Source: CAD feature listing. Evaluate the final solid. Frame: model axes, mm. A direction names the side the tool comes from. Round coordinates to 2 decimals unless told otherwise and drop trailing zeros. Order: outer loops, then holes, each group sorted by start corner. A loop starts at its lowest first (then second) coordinate and runs counter-clockwise, first axis right, second up. Notation, with made-up numbers: (34.5, -4) - (43.5, -4) arc R28 ccw to (43.5, 16) - close; hole circle Ø7 at (69, 59.5). An arc over 180 degrees is marked (long way). Use one line per item in the form item = value. Start each with the question number.
Q1. Cut plane C-C, the plane y = -1.25. Give the number of separate pieces and of enclosed holes in the cut face, and give its area (3 significant figures).
Q2. Cut plane A-A, the plane z = 3.5. Return the cut outline in (x, y), and give its area (3 significant figures).
Q3. Cut plane B-B, the plane x = -13. Return the cut outline in (y, z), and give its area (3 significant figures).
Q4. Ray query, line 1 (X direction, y = -2, z = 3); line 2 (Z direction, x = -2.5, y = -6.75); line 3 (X direction, y = -5.25, z = 1). Return the intervals inside material, ascending. Write a range as [from, to].
Q5. Set-up query: faces 1 (the cylindrical face through (11.616, -1.252, 3.556)), 2 (the cylindrical face through (0.18, -8.38, 4.16)), 3 (the cylindrical face through (-10.57, -5.47, 6.05)), 4 (the cylindrical face through (10.58, -5.47, 0.32)). Return all of +Z, -Z, +X, -X, +Y, -Y with unobstructed straight access to the full face (end or side cutting, diameter ignored); none if empty.
Q6. Cut plane D-D, the plane x = -7. Return the cut outline in (y, z).
Q7. Draft query along X for faces 5 (the cylindrical face through (-9.525, -5.67, 3.211)), 6 (the flat face through (-14.2, -2.54, 2.5)), 7 (the cylindrical face through (0.131, -5.968, 1.002)). Return one class per face: released by +X, released by -X, zero draft, split by the parting line, or undercut.
Q8. Pin query (flat end, axial travel): pin 1 Ø1.5 at (y, z) = (-3.5, 4.5) entering from -X; pin 2 Ø2 at (x, z) = (-12.827, 3.175) entering from -Y; pin 3 Ø3 at (y, z) = (-8.5, 3.5) entering from -X; pin 4 Ø4 at (x, y) = (2, -5.5) entering from +Z. Return the tip coordinate at first contact, or that it passes through.
from build123d import *

# Parameters (mm, degrees)
F1_DEPTH = 6.35
F2_DEPTH = 2.54
F3_R     = 1.27
F4_DEPTH = 25.4
F7_DEPTH = 10.16
F8_R     = 0.508
F9_SIZE  = 0.508


with BuildPart() as f1:
    # F0 (on Top) → F1 (new body)
    with BuildSketch(Plane.XY):
        with BuildLine():
            ThreePointArc((8.382, 0), (0, -8.382), (-8.382, 0))
            Line((-8.382, 0), (-17.272, 0))
            Line((-17.272, 0), (-17.272, -2.54))
            Line((-17.272, -2.54), (-15.24, -2.54))
            ThreePointArc((-15.24, -2.54), (-8.8418597658, -9.1442704985), (0, -11.6689691252))
            ThreePointArc((0, -11.6689691252), (8.8418597658, -9.1442704985), (15.24, -2.54))
            Line((15.24, -2.54), (17.272, -2.54))
            Line((17.272, -2.54), (17.272, 0))
            Line((17.272, 0), (8.382, 0))
        make_face()
    extrude(amount=F1_DEPTH)

    # F0 (on Top) → F2 (join)
    with BuildSketch(Plane.XY):
        with BuildLine():
            ThreePointArc((5.969, 0), (0, -5.969), (-5.969, 0))
            Line((-5.969, 0), (-8.382, 0))
            ThreePointArc((-8.382, 0), (0, -8.382), (8.382, 0))
            Line((8.382, 0), (5.969, 0))
        make_face()
    extrude(amount=F2_DEPTH)

    # F3 (on face) → F4 (cut)
    with BuildSketch(Plane(origin=(0, 0, 0), x_dir=(-1, 0, 0), z_dir=(0, 1, 0))):
        with Locations((-12.827, 3.175)):
            Circle(F3_R)
        with Locations((12.827, 3.175)):
            Circle(F3_R)
    extrude(amount=-F4_DEPTH, mode=Mode.SUBTRACT)

    # F6 (on offset) → F7 (cut)
    with BuildSketch(Plane(origin=(0, -12.7, 0), x_dir=(-1, 0, 0), z_dir=(0, 1, 0))):
        with BuildLine():
            ThreePointArc((12.7267177602, -0.1254768553), (15.1261381042, 0.8049434652), (16.129, 3.175))
            ThreePointArc((16.129, 3.175), (15.1883800681, 5.483048564), (12.9024172176, 6.4761386283))
            ThreePointArc((12.9024172176, 6.4761386283), (9.5261688447, 3.2628503518), (12.7267177602, -0.1254768553))
        make_face()
        with BuildLine():
            ThreePointArc((-12.7793536698, -0.1266562249), (-10.4753482207, 0.8570401408), (-9.525, 3.175))
            ThreePointArc((-9.525, 3.175), (-10.4531379965, 5.4702087461), (-12.7157832758, 6.4751264885))
            ThreePointArc((-12.7157832758, 6.4751264885), (-16.128846925, 3.2067943984), (-12.7793536698, -0.1266562249))
        make_face()
        with BuildLine():
            ThreePointArc((-12.7793536698, -0.1266562249), (-16.128846925, 3.2067943984), (-12.7157832758, 6.4751264885))
            Line((-12.7157832758, 6.4751264885), (-20.0003515929, 7.2803031653))
            Line((-20.0003515929, 7.2803031653), (-20.0003515929, -2.0043456461))
            Line((-20.0003515929, -2.0043456461), (-12.7793536698, -0.1266562249))
        make_face()
        with BuildLine():
            ThreePointArc((12.9024172176, 6.4761386283), (15.1883800681, 5.483048564), (16.129, 3.175))
            ThreePointArc((16.129, 3.175), (15.1261381042, 0.8049434652), (12.7267177602, -0.1254768553))
            Line((12.7267177602, -0.1254768553), (20.6403024495, -1.1550099589))
            Line((20.6403024495, -1.1550099589), (20.6403024495, 7.2800177149))
            Line((20.6403024495, 7.2800177149), (12.9024172176, 6.4761386283))
        make_face()
    extrude(amount=F7_DEPTH, mode=Mode.SUBTRACT)

    # F8
    f8_edges = [f1.edges().sort_by_distance(p)[0] for p in [
        (-11.920039, -4.675696, 6.35),
        (-11.920039, -4.675696, 0),
        (11.920039, -4.675696, 6.35),
        (11.920039, -4.675696, 0),
    ]]
    fillet(f8_edges, radius=F8_R)

    # F9
    f9_edges = [f1.edges().sort_by_distance(p)[0] for p in [
        (0, -5.969, 2.54),
        (7.1755, 0, 2.54),
        (-7.1755, 0, 2.54),
    ]]
    chamfer(f9_edges, length=F9_SIZE)


solid = f1.part
Completed:
q1.separate_pieces = 2
q1.enclosed_holes = 2
q1.area = 116 mm2
q2.outline = (-17.27, -2.54) - (-14.05, -2.54) - (-14.05, 0) - (-17.27, 0) - close; (-11.6, -2.54) - (-9.54, -2.54) - (-9.54, -8.7) arc R17.78 ccw to (0, -11.67) arc R17.78 ccw to (9.54, -8.7) - (9.54, -2.54) - (11.6, -2.54) - (11.6, 0) - (8.38, 0) arc R8.38 cw to (-8.38, 0) - (-11.6, 0) - close; (14.05, -2.54) - (17.27, -2.54) - (17.27, 0) - (14.05, 0) - close
q2.area = 120 mm2
q3.outline = (-2.54, 0) - (0, 0) - (0, 1.92) - (-2.54, 1.92) - close; (-2.54, 4.43) - (0, 4.43) - (0, 6.35) - (-2.54, 6.35) - close
q3.area = 9.74 mm2
q4.line_1 = [-17.27, -14.08], [-11.57, -8.14], [8.14, 11.57], [14.08, 17.27]
q4.line_2 = [0, 2.54]
q4.line_3 = [-10.34, -2.84], [2.84, 10.34]
q5.face_1 = +Y, -Y
q5.face_2 = +Z, +Y
q5.face_3 = -X, -Y
q5.face_4 = +X, -Y
q6.outline = (-10.11, 0) - (0, 0) - (0, 2.03) - (-0.51, 2.54) - (-4.61, 2.54) - (-4.61, 6.35) - (-10.11, 6.35) - close
q7.face_5 = released by -X
q7.face_6 = zero draft
q7.face_7 = undercut
q8.pin_1 = -10.26
q8.pin_2 = through
q8.pin_3 = -10.07
q8.pin_4 = 2.54
